Answer from the drawing. Dimensions are ordinates in mm from the lowest x, y and z of the part. A direction names the side the tool comes from. Coordinates: 2 decimals unless noted, no trailing zeros. Order: outer loops, then holes, each group sorted by start corner. A loop starts at its lowest first (then second) coordinate and runs counter-clockwise, first axis right, second up.
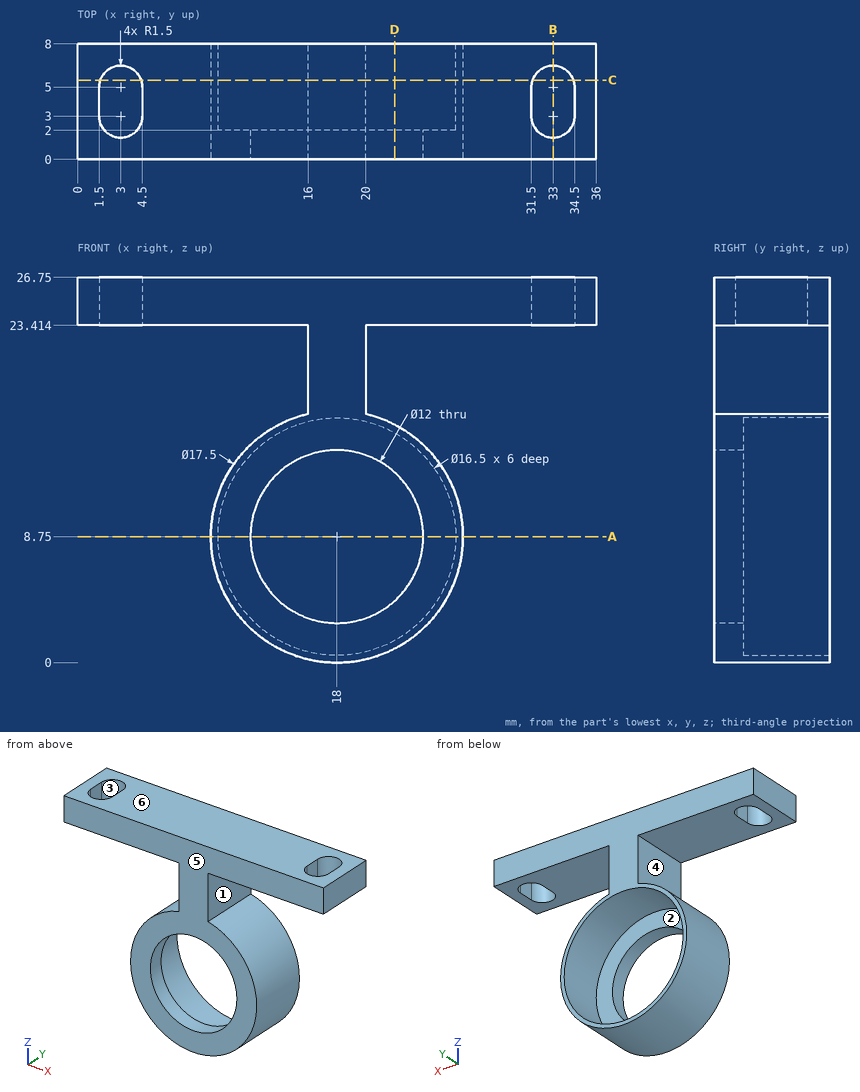
1. The part is cut by section B-B (x = 33). Determine the outline of the cut face in (y, z), plus the area to 3 significant figures.
2. The part is cut by section D-D (x = 22). Determine the outline of the cut face in (y, z), plus the area to 3 significant figures.
3. Flat-ended cylindrical pins translate along their axes: pin 1 (2.5 mm diameter, centred on x = 11, y = 6, fed in from -Z) (1 decimal); pin 2 (3 mm diameter, centred on y = 5, z = 19, fed in from +X); pin 3 (4 mm diameter, centred on x = 30.5, y = 2.5, fed in from -Z). Find the tip coordinate at first contact, or state that the pin passes through.
4. The mould has two halves that part along Z. Classify the marked faces 4, 5 and 6: released by +Z, released by -Z, zero draft, split by the parting line, or undercut.
5. The part is cut by section A-A (z = 8.75). Determine the outline of the cut face in (x, y), plus the area to 3 significant figures.
6. The part is cut by section C-C (y = 5.5). Determine the outline of the cut face in (x, z), plus the area to 3 significant figures.
7. For the marked faces 1, 2 and 3, determine the directions among +Z, -Z, +X, -X, +Y, -Y from which every point of the face is accessible in a straight line to the end or side of a thin tool.
8. Consider probe 1 along X at (y, z) = (3, 24.75); probe 2 along Z at (x, y) = (18, 0.55); probe 3 along X at (y, z) = (1, 8.5) (1 decimal). Determine where each line is inside the solid, lowest interval first.
Worked out:
1. outline: (0, 23.41) - (1.5, 23.41) - (1.5, 26.75) - (0, 26.75) - close; (6.5, 23.41) - (8, 23.41) - (8, 26.75) - (6.5, 26.75) - close
1. area: 10.0 mm2
2. outline: (0, 0.97) - (8, 0.97) - (8, 1.53) - (2, 1.53) - (2, 4.28) - (0, 4.28) - close; (0, 13.22) - (2, 13.22) - (2, 15.97) - (8, 15.97) - (8, 16.53) - (0, 16.53) - close; (0, 23.41) - (8, 23.41) - (8, 26.75) - (0, 26.75) - close
2. area: 46.7 mm2
3. pin 1: stops at z = 2.2
3. pin 2: stops at x = 20
3. pin 3: stops at z = 23.41
4. face 4: undercut
4. face 5: zero draft
4. face 6: released by +Z
5. outline: (9.25, 0) - (12, 0) - (12, 2) - (9.75, 2) - (9.75, 8) - (9.25, 8) - close; (24, 0) - (26.75, 0) - (26.75, 8) - (26.25, 8) - (26.25, 2) - (24, 2) - close
5. area: 17.0 mm2
6. outline: (0, 23.41) - (1.59, 23.41) - (1.59, 26.75) - (0, 26.75) - close; (4.41, 23.41) - (16, 23.41) - (16, 17.27) arc R8.75 ccw (long way) to (20, 17.27) - (20, 23.41) - (31.59, 23.41) - (31.59, 26.75) - (4.41, 26.75) - close; (34.41, 23.41) - (36, 23.41) - (36, 26.75) - (34.41, 26.75) - close; hole circle Ø16.5 at (18, 8.75)
6. area: 152 mm2
7. face 1: +X, +Y, -Y
7. face 2: +Y
7. face 3: +Z, -Z
8. probe 1: x = 0 to 1.5, 4.5 to 31.5, 34.5 to 36
8. probe 2: z = 0 to 2.75, 14.75 to 26.75
8. probe 3: x = 9.3 to 12, 24 to 26.7
